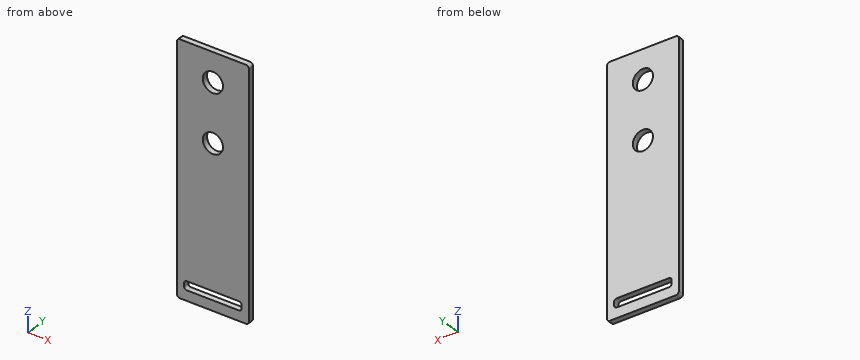
from build123d import *

# Parameters (mm, degrees)
F0_R     = 3.5
F1_DEPTH = 2


with BuildPart() as f1:
    # F0 (on Front) → F1 (new body)
    with BuildSketch(Plane.XZ):
        with BuildLine():
            Line((-11.5, -42.5), (11.5, -42.5))
            ThreePointArc((11.5, -42.5), (12.207107, -42.207107), (12.5, -41.5))
            Line((12.5, -41.5), (12.5, 41.5))
            ThreePointArc((12.5, 41.5), (12.207107, 42.207107), (11.5, 42.5))
            Line((11.5, 42.5), (-11.5, 42.5))
            ThreePointArc((-11.5, 42.5), (-12.207107, 42.207107), (-12.5, 41.5))
            Line((-12.5, 41.5), (-12.5, -41.5))
            ThreePointArc((-12.5, -41.5), (-12.207107, -42.207107), (-11.5, -42.5))
        make_face()
        with BuildLine():
            ThreePointArc((10, -38), (9.707107, -38.707107), (9, -39))
            Line((9, -39), (-9, -39))
            ThreePointArc((-9, -39), (-9.707107, -38.707107), (-10, -38))
            Line((-10, -38), (-10, -37))
            ThreePointArc((-10, -37), (-9.707107, -36.292893), (-9, -36))
            Line((-9, -36), (9, -36))
            ThreePointArc((9, -36), (9.707107, -36.292893), (10, -37))
            Line((10, -37), (10, -38))
        make_face(mode=Mode.SUBTRACT)
        with Locations((0, 12.5)):
            Circle(F0_R, mode=Mode.SUBTRACT)
        with Locations((0, 32.5)):
            Circle(F0_R, mode=Mode.SUBTRACT)
    extrude(amount=F1_DEPTH)


solid = f1.part
Model file for the job. Use its own axes, mm. Give positions to 0.01 mm unless a question says otherwise; leave off trailing zeros. Order: outer loops, then holes, each group sorted by start corner. A loop starts at its lowest first (then second) coordinate and runs counter-clockwise, first axis right, second up. Notation, with made-up numbers: (29.5, 84.25) - (49.5, 84.25) arc R15 ccw to (49.5, 100.25) - close; hole circle Ø5 at (65.25, -19). An arc over 180 degrees is marked (long way). Write item = value, one per line. Start each with the question number.
1. Cut at B-B, the plane x = 0. List the corners of the cut face in (y, z), and give its area (3 significant figures).
2. Probe line 1 along Z through (x, y) = (0, -0.85); line 2 along Z through (x, y) = (5, -0.75); line 3 along X through (y, z) = (-1.4, -37.5). List the from-to ranges inside material, lowest first.
3. Cut at A-A, the plane z = 12.5. List the corners of the cut face in (x, y).
4. Cut at D-D, the plane x = -7.25. List the corners of the cut face in (y, z).
5. Cut at C-C, the plane y = -1. List the corners of the cut face in (x, z).
Taken from the geometry:
q1.outline = (-2, -42.5) - (0, -42.5) - (0, -39) - (-2, -39) - close; (-2, -36) - (0, -36) - (0, 9) - (-2, 9) - close; (-2, 16) - (0, 16) - (0, 29) - (-2, 29) - close; (-2, 36) - (0, 36) - (0, 42.5) - (-2, 42.5) - close
q1.area = 136 mm²
q2.line_1 = -42.5 to -39, -36 to 9, 16 to 29, 36 to 42.5
q2.line_2 = -42.5 to -39, -36 to 42.5
q2.line_3 = -12.5 to -10, 10 to 12.5
q3.outline = (-12.5, -2) - (-3.5, -2) - (-3.5, 0) - (-12.5, 0) - close; (3.5, -2) - (12.5, -2) - (12.5, 0) - (3.5, 0) - close
q4.outline = (-2, -42.5) - (0, -42.5) - (0, -39) - (-2, -39) - close; (-2, -36) - (0, -36) - (0, 42.5) - (-2, 42.5) - close
q5.outline = (-12.5, -41.5) arc R1 ccw to (-11.5, -42.5) - (11.5, -42.5) arc R1 ccw to (12.5, -41.5) - (12.5, 41.5) arc R1 ccw to (11.5, 42.5) - (-11.5, 42.5) arc R1 ccw to (-12.5, 41.5) - close; hole (-10, -38) arc R1 ccw to (-9, -39) - (9, -39) arc R1 ccw to (10, -38) - (10, -37) arc R1 ccw to (9, -36) - (-9, -36) arc R1 ccw to (-10, -37) - close; hole circle Ø7 at (0, 12.5); hole circle Ø7 at (0, 32.5)
